Autodesk Fusion 360 part; units mm, degrees
box "BoxPrimitive1" add length 100 width 200 height 60 placed x (0, 0, 1) y (1, 0, 0) z (0, 1, 0) at (-155.2109, 0, -8.8747)
hole "Hole1" at (-125.851, 60, 40.8743) direction (0, -1, 0) diameter 16 depth 100 tip angle 118
sketch "Sketch7" plane through (0, 0, 0) normal (0, -1, 0) x (1, 0, 0)
  circle A0 centre (-125.851, 40.8743) radius 8
  line L0 (44.7891, 91.1253) -> (-155.2109, 91.1253)
  line L1 (-155.2109, 91.1253) -> (-155.2109, -8.8747)
  line L2 (-155.2109, -8.8747) -> (44.7891, -8.8747)
  line L3 (44.7891, -8.8747) -> (44.7891, 91.1253)
  line L4 (-33.4877, 55.3548) -> (8.1123, 55.3548)
  line L5 (8.1123, 55.3548) -> (8.1123, 13.7548)
  line L6 (8.1123, 13.7548) -> (-33.4877, 13.7548)
  line L7 (-33.4877, 13.7548) -> (-33.4877, 55.3548)
  dimension "d9" = 41.6
  dimension "d10" = 41.6
extrude "Extrude1" cut sketch "Sketch7" against normal blind 60 contours L4 L5 L6 L7
Build history of the part. All positions in model axes, mm. A direction names the side the tool comes from. Coordinates: 2 decimals unless noted, no trailing zeros. Order: outer loops, then holes, each group sorted by start corner. A loop starts at its lowest first (then second) coordinate and runs counter-clockwise, first axis right, second up. Notation, with made-up numbers: (-23, 83.5) - (-8, 83.5) arc R13 ccw to (-8, 87.5) - close; hole circle Ø9 at (-19, 22). An arc over 180 degrees is marked (long way). Write item = value, one per line. Start each with the question number.
1) Saw through at C-C on x = -131. Write the cut outline in (y, z), then the cut area to 3 significant figures.
2) Saw through at B-B on z = 43. Write the cut outline in (x, y), then the cut area to 3 significant figures.
3) Two-plate mould, pull along Z, no slides. Class faces 3 (the face through (-33.488, 30, 34)), 4 (the face through (-57, 30, 91.125)), 5 (the face through (44.789, 30, 42)): pulls with the +Z half, pulls with the -Z half, needs draft (parallel to the pull), parting line crosses it, or undercut.
4) Saw through at D-D on y = 29. Write the cut outline in (x, z), then the cut area to 3 significant figures.
5) Wall check: line 1 along Z through (x, y) = (-23, 54.5); line 2 along X through (y, z) = (17.5, 33.5); line 3 along X through (y, z) = (24, 32). Give the ranges that are in metal, low to high. Write a range as from..to.
6) Saw through at A-A on z = 25.5. Write the cut outline in (x, y), then the cut area to 3 significant figures.
7) 3-axis set-ups, long thin cutter, end or side, ignore diameter. For faces 1 (the face through (-54, 60, 40)), 2 (the face through (-13, 30, 55.355)): which of +Z, -Z, +X, -X, +Y, -Y reach the whole face in a straight line?
From the geometry:
q1.outline = (0, -8.87) - (60, -8.87) - (60, 34.75) - (0, 34.75) - close; (0, 47) - (60, 47) - (60, 91.13) - (0, 91.13) - close
q1.area = 5,270 mm^2
q2.outline = (-155.21, 0) - (-133.56, 0) - (-133.56, 60) - (-155.21, 60) - close; (-118.14, 0) - (-33.49, 0) - (-33.49, 60) - (-118.14, 60) - close; (8.11, 0) - (44.79, 0) - (44.79, 60) - (8.11, 60) - close
q2.area = 8,580 mm^2
q3.face_3 = undercut
q3.face_4 = pulls with the +Z half
q3.face_5 = needs draft
q4.outline = (-155.21, -8.87) - (44.79, -8.87) - (44.79, 91.13) - (-155.21, 91.13) - close; hole circle Ø16 at (-125.85, 40.87); hole (-33.49, 13.75) - (8.11, 13.75) - (8.11, 55.35) - (-33.49, 55.35) - close
q4.area = 18,100 mm^2
q5.line_1 = -8.87..13.75, 55.35..91.13
q5.line_2 = -155.21..-128.95, -122.75..-33.49, 8.11..44.79
q5.line_3 = -155.21..-33.49, 8.11..44.79
q6.outline = (-155.21, 0) - (-33.49, 0) - (-33.49, 60) - (-155.21, 60) - close; (8.11, 0) - (44.79, 0) - (44.79, 60) - (8.11, 60) - close
q6.area = 9,500 mm^2
q7.face_1 = +Z, -Z, +X, -X, +Y
q7.face_2 = +Y, -Y
